from build123d import *

# Parameters (mm, degrees)
SKETCH_1_R          = 4.5
EXTRUDE_1_DEPTH     = 1
SKETCH_2_R          = 2
EXTRUDE_2_DEPTH     = 15
CUT_EXTRUDE_1_DEPTH = 1


with BuildPart() as part:
    # 草图1 → 凸台-拉伸1 (new body)
    with BuildSketch(Plane(origin=(0, 0, 0), x_dir=(1, 0, 0), z_dir=(0, 1, 0))):
        Circle(SKETCH_1_R)
    extrude(amount=EXTRUDE_1_DEPTH)

    # 草图2 → 凸台-拉伸2 (add)
    with BuildSketch(Plane.XZ):
        Circle(SKETCH_2_R)
    extrude(amount=EXTRUDE_2_DEPTH)

    # 草图3 → 切除-旋转2 (revolve, cut)
    with BuildSketch(Plane.XY):
        with BuildLine():
            ThreePointArc((5.590055425, 0.474587026), (2.807346543, 0.868357929), (0, 1))
            Line((0, 1), (0, 3.329372604))
            Line((0, 3.329372604), (5.734393967, 3.279293278))
            Line((5.734393967, 3.279293278), (5.590055425, 0.474587026))
        make_face()
    revolve(axis=Axis((0, 0, 0), (0, 1, 0)), mode=Mode.SUBTRACT)

    # 草图4 → 切除-拉伸1 (cut)
    with BuildSketch(Plane.XZ):
        Polygon((0, -1.802383699), (1.56091007, -0.901191849), (1.56091007, 0.901191849), (0, 1.802383699), (-1.56091007, 0.901191849), (-1.56091007, -0.901191849), align=None)
    extrude(amount=-CUT_EXTRUDE_1_DEPTH, mode=Mode.SUBTRACT)


solid = part.part
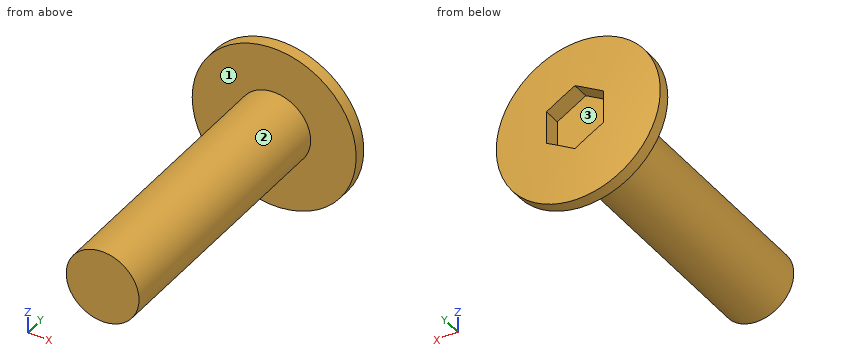
Verification items for the finished model (mm, model axes). Face numbers are marked on the shaded views. Coordinates: 2 decimals unless noted, no trailing zeros. Write each loop counter-clockwise with the first axis right and the second up, starting at its lowest first coordinate (ties: lowest second). Pieces come first, ordered by that corner, then holes. Notation, with made-up numbers: (5.25, 85) - (57.25, 85) arc R29 cw to (57.25, 113) - close; hole circle Ø9 at (17, 89.25). An arc over 180 degrees is marked (long way). Answer as a JSON object with one key per item and string values.
(1) Thickness scan on line 1 along Z through (x, y) = (-1.25, -6.5); line 2 along Y through (x, z) = (1, 0.5); line 3 along Y through (x, z) = (1.5, 4). Record the ranges inside material, lowest first.
Report:
{"line 1": "-1.56 to 1.56", "line 2": "-15 to 0", "line 3": "0 to 0.69"}
(2) Cross-section at A-A on z = 0. Record the cut outline in (x, y), plus the area to 3 significant figures.
Report:
{"outline": "(-4.5, 0) - (-2, 0) - (-2, -15) - (2, -15) - (2, 0) - (4.5, 0) - (4.5, 0.66) arc R30 ccw to (1.56, 0.96) - (1.56, 0) - (-1.56, 0) - (-1.56, 0.96) arc R30 ccw to (-4.5, 0.66) - close", "area": "64.9 mm^2"}
(3) Mould release check, pull along X, two halves, no side actions. Record for the marked faces 1, 2 and 3: pulls with the +X half, pulls with the -X half, needs draft (parallel to the pull), parting line crosses it, or undercut.
Report:
{"face 1": "needs draft", "face 2": "parting line crosses it", "face 3": "undercut"}
(4) Gauge pin test, flat ends, axial feed: pin 1 Ø1 at (y, z) = (-2, 2) entering from +X; pin 2 Ø3 at (x, y) = (0.5, -13) entering from +Z; pin 3 Ø4 at (y, z) = (-9, 1) entering from -X. Record the tip position at first contact, or that the pin passes through.
Report:
{"pin 1": "x = 1.32", "pin 2": "z = 2", "pin 3": "x = -2"}
(5) Cross-section at D-D on x = 3.5. Record the cut outline in (y, z), plus the area to 3 significant figures.
Report:
{"outline": "(0, -2.83) - (0.66, -2.83) arc R29.8 ccw to (0.66, 2.83) - (0, 2.83) - close", "area": "4.24 mm^2"}
(6) Cross-section at B-B on x = -1. Record the cut outline in (y, z), plus the area to 3 significant figures.
Report:
{"outline": "(-15, -1.73) - (0, -1.73) - (0, -4.39) - (0.66, -4.39) arc R29.98 ccw to (0.96, -1.23) - (0, -1.23) - (0, 1.23) - (0.96, 1.23) arc R29.98 ccw to (0.66, 4.39) - (0, 4.39) - (0, 1.73) - (-15, 1.73) - close", "area": "57.3 mm^2"}
(7) Cross-section at C-C on y = -1. Record the cut outline in (x, z).
Report:
{"outline": "circle Ø4 at (0, 0)"}
